Part model, mm, in its own coordinate system. A direction names the side the tool comes from. Coordinates: 2 decimals unless noted, no trailing zeros. Loops run counter-clockwise (first coordinate to the right, second up) from the corner with the lowest first, then second, coordinate; pieces in that order, holes last. Notation, with made-up numbers: (7, 56.5) - (59, 56.5) arc R19 cw to (59, 78.5) - close; hole circle Ø10 at (40, -16). An arc over 180 degrees is marked (long way). Answer as CSV lines item,"result".
Autodesk Inventor part; units mm, degrees
ref_plane "YZ Plane" through (0, 0, 0) normal (1, 0, 0) x (0, 1, 0)
ref_plane "XZ Plane" through (0, 0, 0) normal (0, 1, 0) x (-1, 0, 0)
ref_plane "XY Plane" through (0, 0, 0) normal (0, 0, 1) x (1, 0, 0)
sketch "Sketch1" plane through (0, 0, 0) normal (0, 1, 0) x (-1, 0, 0)
  line L0 (0, 0) -> (2, 0)
  line L1 (2, 0) -> (2, -8.7)
  line L2 (2, -8.7) -> (5, -8.7)
  line L3 (5, -8.7) -> (0, -15)
  line L4 (0, -15) -> (0, 0)
  dimension "d0" = 15
  dimension "d1" = 5
  dimension "d3" = 2
  dimension "d5" = 8.7
revolve "Revolution1" add sketch "Sketch1" angle 360 about axis through (0, 0, -15) along (0, 0, 1)
sketch "Sketch2" plane through (0, 0, -8.7) normal (0, 0, 1) x (1, 0, 0)
  circle A0 centre (0, 0) radius 2
  circle A1 centre (0, 0) radius 5
  line L0 (1.7321, 1) -> (4.899, 1)
  line L1 (0, 0) -> (5, 0) construction
  line L2 (1.7321, -1) -> (4.899, -1)
  line L3 (-1, 1.7321) -> (-1, 4.899)
  line L4 (1, 1.7321) -> (1, 4.899)
  line L5 (-1.7321, -1) -> (-4.899, -1)
  line L6 (-1.7321, 1) -> (-4.899, 1)
  line L7 (1, -1.7321) -> (1, -4.899)
  line L8 (-1, -1.7321) -> (-1, -4.899)
  dimension "d8" = 1
  dimension "d11" = 360
extrude "Extrusion1" add sketch "Sketch2" along normal blind 2.5 contours A0 L0 A1 L2 | A0 L3 A1 L4 | L7 A1 L8 A0 | A0 L5 A1 L6
properties part number "Goma tacómetro"
Q1. Saw through at A-A (z = -7). Give the cut face in (x, y), then the cut area to 3 significant figures.
Results:
outline,"(-4.9, -1) - (-1.73, -1) arc R2 ccw to (-1, -1.73) - (-1, -4.9) arc R5 ccw to (1, -4.9) - (1, -1.73) arc R2 ccw to (1.73, -1) - (4.9, -1) arc R5 ccw to (4.9, 1) - (1.73, 1) arc R2 ccw to (1, 1.73) - (1, 4.9) arc R5 ccw to (-1, 4.9) - (-1, 1.73) arc R2 ccw to (-1.73, 1) - (-4.9, 1) arc R5 ccw to start"
area,"37.0 mm^2"
Q2. Which spindle directions (+Z, -Z, +X, -X, +Y, -Y) get a long thin tool onto all of the face, cutting with end or side? Do faces 1 (the face through (1.474, 1.352, -3.444)), 2 (the face through (3, 1, -7)), 3 (the face through (-2, 2, -8.7)). Say none if no direction does.
Results:
face 1,"+Z"
face 2,"+Z, +X, +Y"
face 3,"+Z, -X, +Y"
Q3. Wall check: L1, parallel to X at y = -4.5, z = -8.5; L2, parallel to X at y = 0, z = -3.5. Give the ranges that are in metal, low to high.
Results:
L1,"x = -1 to 1"
L2,"x = -2 to 2"
Q4. Flat gauge pins, fed straight in: pin 1 (2.5 mm diameter, centred on y = 2.5, z = -7, fed in from +X); pin 2 (0.7 mm diameter, centred on x = -3, z = -8, fed in from +Y); pin 3 (0.7 mm diameter, centred on x = 3.5, z = -7.5, fed in from -Y); pin 4 (2 mm diameter, centred on x = 0, y = -0.5, fed in from +Z). Where does each tip first touch, or does it go through?
Results:
pin 1,"stops at x = 1.56"
pin 2,"stops at y = 1"
pin 3,"stops at y = -1"
pin 4,"stops at z = 0"
